Autodesk Inventor part; units mm, degrees
ref_plane "YZ Plane" through (0, 0, 0) normal (1, 0, 0) x (0, 1, 0)
ref_plane "XZ Plane" through (0, 0, 0) normal (0, 1, 0) x (-1, 0, 0)
ref_plane "XY Plane" through (0, 0, 0) normal (0, 0, 1) x (1, 0, 0)
sketch "okrąg" plane through (0, 0, 0) normal (0, 1, 0) x (-1, 0, 0)
  circle A0 centre (0, 0) radius 90
  circle A1 centre (0, 0) radius 97.5
  line L0 (0, 0) -> (0, -95.75) construction
  line L1 (-18.3899, -95.75) -> (18.3899, -95.75)
  line L2 (0, 0) -> (95.75, 0) construction
  line L3 (95.75, -18.3899) -> (95.75, 18.3899)
  line L4 (0, 0) -> (0, 95.75) construction
  line L5 (18.3899, 95.75) -> (-18.3899, 95.75)
  line L6 (0, 0) -> (-95.75, 0) construction
  line L7 (-95.75, 18.3899) -> (-95.75, -18.3899)
  point P0 (-95.75, 18.3899)
  point P1 (-95.75, -18.3899)
  point P2 (-18.3899, -95.75)
  point P3 (95.75, -18.3899)
  point P4 (95.75, 18.3899)
  point P5 (18.3899, 95.75)
  point P6 (-18.3899, 95.75)
  dimension "d1" = 195
  dimension "d0" = 180
  dimension "d2" = 95.75
  dimension "d5" = 360
extrude "Wyciągnięcie proste1" add sketch "okrąg" along normal mid plane 65 contours L3 A1 L1 L7 L5
sketch "podpora" plane through (0, 0, 0) normal (0, 1, 0) x (-1, 0, 0)
  circle A0 centre (0, 0) radius 90
  line L0 (2.5, 0) -> (-2.5, 0) construction
  line L1 (-2.5, -90) -> (-2.5, 90)
  line L2 (2.5, -90) -> (2.5, 90)
  circle A1 centre (0, 0) radius 11.5
  point P0 (-2.5, -11.225)
  point P1 (-2.5, -89.9653)
  point P2 (2.5, -89.9653)
  point P3 (2.5, -11.225)
  point P4 (2.5, 11.225)
  point P5 (2.5, 89.9653)
  point P6 (-2.5, 89.9653)
  point P7 (-2.5, 11.225)
  dimension "d12" = 180
  dimension "d13" = 5
  dimension "d14" = 180
  dimension "d15" = 180
  dimension "d16" = 23
extrude "Wyciągnięcie proste2" add sketch "podpora" along normal mid plane 3 contours L2 A1 L1 A0 | A0 L1 A1 L2 | A1 L2 | L2 A1 L1 | L1 A1
sketch "Szkic5" plane through (-18.3899, 32.5, 95.75) normal (0, 0, 1) x (1, 0, 0)
  line L0 (0, 0) -> (18.3899, 0) construction
  line L1 (18.3899, 0) -> (18.3899, -15) construction
  line L2 (18.3899, -15) -> (18.3899, -50) construction
  circle A0 centre (18.3899, -15) radius 1.5
  circle A1 centre (18.3899, -50) radius 1.5
  point P0 (18.3899, -32.5)
  dimension "d28" = 18.3899
  dimension "d32" = 32.5
  dimension "d33" = 32.5
  dimension "d34" = 15
  dimension "d35" = 35
  dimension "d36" = 3
  dimension "d37" = 3
extrude "Wyciągnięcie proste4" cut sketch "Szkic5" against normal through all
sketch "Szkic6" plane through (-95.75, -32.5, 18.3899) normal (-1, 0, 0) x (0, 0, 1)
  line L0 (-18.3899, 32.5) -> (-18.3899, 50) construction
  line L1 (-18.3899, 32.5) -> (-18.3899, 15) construction
  circle A0 centre (-18.3899, 15) radius 1.5
  circle A1 centre (-18.3899, 50) radius 1.5
  dimension "d40" = 17.5
  dimension "d41" = 17.5
  dimension "d42" = 3
  dimension "d43" = 3
extrude "Wyciągnięcie proste5" cut sketch "Szkic6" against normal through all
sketch "Szkic7" plane through (18.3899, 32.5, -95.75) normal (0, 0, -1) x (-1, 0, 0)
  line L0 (18.3899, -31) -> (18.3899, -34) construction
  line L1 (15.8899, -31) -> (20.8899, -31)
  line L2 (20.8899, -31) -> (20.8899, -28)
  line L3 (20.8899, -28) -> (15.8899, -28)
  line L4 (15.8899, -28) -> (15.8899, -31)
  line L5 (15.8899, -34) -> (20.8899, -34)
  line L6 (20.8899, -34) -> (20.8899, -37)
  line L7 (20.8899, -37) -> (15.8899, -37)
  line L8 (15.8899, -37) -> (15.8899, -34)
  point P0 (18.3899, -32.5)
  dimension "d46" = 3
  dimension "d47" = 5
  dimension "d48" = 3
  dimension "d49" = 3
  dimension "d50" = 5
extrude "Wyciągnięcie proste6" cut sketch "Szkic7" against normal through all
equation "\"d12\" = d0"
equation "\"d14\" = d0"
equation "\"d15\" = d0"
properties part number "001-001"
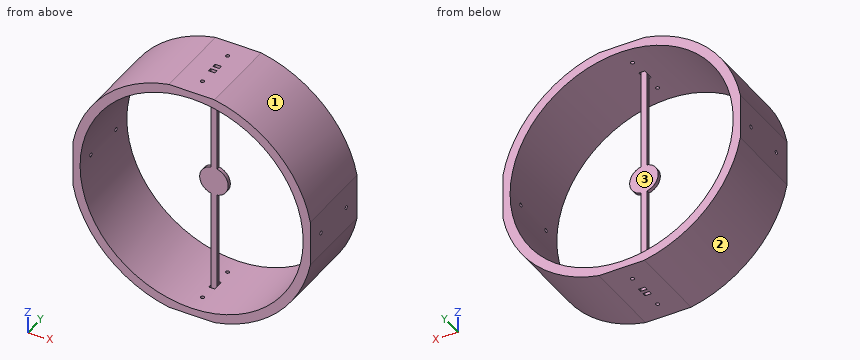
Could you check a few things on this model? Use its own coordinates, in mm. Face numbers are marked on the shaded views. Give positions to 0.01 mm unless a question says otherwise; leave off trailing zeros. Order: outer loops, then holes, each group sorted by start corner. A loop starts at its lowest first (then second) coordinate and runs counter-clockwise, first axis right, second up. Notation, with made-up numbers: (86, 72) -> (121, 72) arc R35 ccw to (121, 106) -> close; hole circle Ø3 at (-39, 88.25). An arc over 180 degrees is marked (long way). Return JSON: item names as keys, results as strings.
1. Imagine slicing it at B-B on y = 24.5. List the corners of the cut face in (x, z) for me, then the cut area to 3 significant figures.
Answer list:
{"outline": "(-95.75, -18.39) arc R97.5 ccw to (-18.39, -95.75) -> (18.39, -95.75) arc R97.5 ccw to (95.75, -18.39) -> (95.75, 18.39) arc R97.5 ccw to (18.39, 95.75) -> (-18.39, 95.75) arc R97.5 ccw to (-95.75, 18.39) -> close; hole circle Ø180 at (0, 0)", "area": "4,250 mm2"}
2. I need wall thicknesses on line 1 (Y direction, x = 0, z = -92.9); line 2 (Y direction, x = 91.3, z = 0); line 3 (X direction, y = 1, z = -42). Which ranges of each line are inside material? Lowest first, please. Write a range as from..to.
Answer list:
{"line 1": "y = -32.5..-19, -16..-4.5, -1.5..1.5, 4.5..16, 19..32.5", "line 2": "y = -32.5..-19, -16..16, 19..32.5", "line 3": "x = -87.99..-79.6, -2.5..2.5, 79.6..87.99"}
3. Imagine slicing it at C-C on z = 68.5. List the corners of the cut face in (x, y) for me, then the cut area to 3 significant figures.
Answer list:
{"outline": "(-69.38, -32.5) -> (-58.38, -32.5) -> (-58.38, 32.5) -> (-69.38, 32.5) -> close; (-2.5, -1.5) -> (2.5, -1.5) -> (2.5, 1.5) -> (-2.5, 1.5) -> close; (58.38, -32.5) -> (69.38, -32.5) -> (69.38, 32.5) -> (58.38, 32.5) -> close", "area": "1,450 mm2"}
4. For pin 1 Ø3.5 at (y, z) = (-0.5, -68) entering from +X; pin 2 Ø1.5 at (y, z) = (-24.5, 34.5) entering from +X; pin 3 Ø1.8 at (x, y) = (0, -17.5) entering from +Z; pin 4 Ø0.9 at (y, z) = (0.5, 58) entering from +X, each with a flat end and sliding along its axis, tell me the tip position at first contact or that it passes through.
Answer list:
{"pin 1": "stops at x = 71.53", "pin 2": "stops at x = 91.47", "pin 3": "passes through", "pin 4": "stops at x = 78.7"}
5. Thinking about a two-plate mould opening in Z: for the marked faces 1, 2 and 3, which applies, pulls with the +Z half, pulls with the -Z half, needs draft (parallel to the pull), parting line crosses it, or undercut?
Answer list:
{"face 1": "pulls with the +Z half", "face 2": "pulls with the -Z half", "face 3": "undercut"}
6. Imagine slicing it at A-A on x = 46. List the corners of the cut face in (y, z) for me, then the cut area to 3 significant figures.
Answer list:
{"outline": "(-32.5, -85.97) -> (32.5, -85.97) -> (32.5, -77.36) -> (-32.5, -77.36) -> close; (-32.5, 77.36) -> (32.5, 77.36) -> (32.5, 85.97) -> (-32.5, 85.97) -> close", "area": "1,120 mm2"}
7. Imagine slicing it at D-D on x = -48. List the corners of the cut face in (y, z) for me.
Answer list:
{"outline": "(-32.5, -84.87) -> (32.5, -84.87) -> (32.5, -76.13) -> (-32.5, -76.13) -> close; (-32.5, 76.13) -> (32.5, 76.13) -> (32.5, 84.87) -> (-32.5, 84.87) -> close"}
